```python
from build123d import *

# Parameters (mm, degrees)
SKETCH1_W            = 78
SKETCH1_H            = 78
BOSS_EXTRUDE1_DEPTH  = 3
CUT_EXTRUDE1_DEPTH   = 56.235857919
SKETCH3_R            = 1.25
CUT_EXTRUDE2_DEPTH   = 56.235857919
LPATTERN1_COUNT      = 2
LPATTERN1_PITCH      = 30
LPATTERN1_COUNT_DIR2 = 2
LPATTERN1_PITCH_DIR2 = 35


with BuildPart() as part:
    # Sketch1 → Boss-Extrude1 (new body)
    with BuildSketch(Plane.XY):
        Rectangle(SKETCH1_W, SKETCH1_H)
    extrude(amount=BOSS_EXTRUDE1_DEPTH)

    # Sketch2 → Cut-Extrude1 (cut, through all)
    with BuildSketch(Plane(origin=(0, 0, 0), x_dir=(-1, 0, 0), z_dir=(0, 0, -1))):
        with BuildLine():
            Line((-26.5, 27.892304845), (-26.5, 7.107695155))
            ThreePointArc((-26.5, 7.107695155), (-15, 2), (-3.5, 7.107695155))
            Line((-3.5, 7.107695155), (-3.5, 27.892304845))
            ThreePointArc((-3.5, 27.892304845), (-15, 33), (-26.5, 27.892304845))
        make_face()
    cut_extrude1 = extrude(amount=-CUT_EXTRUDE1_DEPTH, mode=Mode.SUBTRACT)

    # Sketch3 → Cut-Extrude2 (cut, through all)
    with BuildSketch(Plane(origin=(0, 0, 0), x_dir=(-1, 0, 0), z_dir=(0, 0, -1))):
        with Locations((-21, 1)):
            Circle(SKETCH3_R)
        with Locations((-9, 34)):
            Circle(SKETCH3_R)
    cut_extrude2 = extrude(amount=-CUT_EXTRUDE2_DEPTH, mode=Mode.SUBTRACT)

    # LPattern1: Cut-Extrude1, Cut-Extrude2 2 × 2
    with Locations(*[(-i * LPATTERN1_PITCH, -j * LPATTERN1_PITCH_DIR2, 0) for i in range(LPATTERN1_COUNT) for j in range(LPATTERN1_COUNT_DIR2) if (i, j) != (0, 0)]):
        add(cut_extrude1, mode=Mode.SUBTRACT)
        add(cut_extrude2, mode=Mode.SUBTRACT)


solid = part.part
```
Could you check a few things on this model? Use its own coordinates, in mm. Round coordinates to 2 decimals unless told otherwise and drop trailing zeros. Loops run counter-clockwise (first coordinate to the right, second up) from the corner with the lowest first, then second, coordinate; pieces in that order, holes last.
Q1. I want a section at D-D (x = 9). Write out the boundary of the cut face in (y, z).
Q2. Please list where these lines run through material, in increasing order: L1, parallel to X at y = -22.5, z = 2.3; L2, parallel to X at y = -5, z = 1.8; L3, parallel to Y at x = 21, z = 2.7.
Q3. I want a section at B-B (x = 24). Write out the boundary of the cut face in (y, z), and give its area (3 significant figures).
Q4. Thinking about a two-plate mould opening in X: for faces 1 (the flat face through (3.5, 17, 1)), 2 (the cylindrical face through (15, 2, 1)), 3 (the flat face through (39, -1, 1)), 4 (the flat face through (-39, -1, 1)), which applies, pulls with the +X half, pulls with the -X half, needs draft (parallel to the pull), parting line crosses it, or undercut?
Q5. I want a section at A-A (y = -9.5). Write out the boundary of the cut face in (x, z).
Q6. I want a section at C-C (z = 0.6). Give the number of separate pieces and of enclosed holes in the cut face, and give its area (3 significant figures).
Answer below:
1. outline: (-39, 0) - (-31.79, 0) - (-31.79, 3) - (-39, 3) - close; (-3.21, 0) - (-2.25, 0) - (-2.25, 3) - (-3.21, 3) - close; (0.25, 0) - (3.21, 0) - (3.21, 3) - (0.25, 3) - close; (31.79, 0) - (32.75, 0) - (32.75, 3) - (31.79, 3) - close; (35.25, 0) - (39, 0) - (39, 3) - (35.25, 3) - close
2. L1: x = -39 to -26.5, -3.5 to 3.5, 26.5 to 39
2. L2: x = -39 to -24.17, -5.83 to 5.83, 24.17 to 39
2. L3: y = -39 to -35.25, -32.75 to -31.79, -3.21 to -0.25, 2.25 to 3.21, 31.79 to 39
3. outline: (-39, 0) - (-30.12, 0) - (-30.12, 3) - (-39, 3) - close; (-4.88, 0) - (4.88, 0) - (4.88, 3) - (-4.88, 3) - close; (30.12, 0) - (39, 0) - (39, 3) - (30.12, 3) - close
3. area: 82.6 mm2
4. face 1: undercut
4. face 2: undercut
4. face 3: pulls with the +X half
4. face 4: pulls with the -X half
5. outline: (-39, 0) - (-26.5, 0) - (-26.5, 3) - (-39, 3) - close; (-3.5, 0) - (3.5, 0) - (3.5, 3) - (-3.5, 3) - close; (26.5, 0) - (39, 0) - (39, 3) - (26.5, 3) - close
6. separate pieces: 1
6. enclosed holes: 12
6. area: 3,480 mm2
